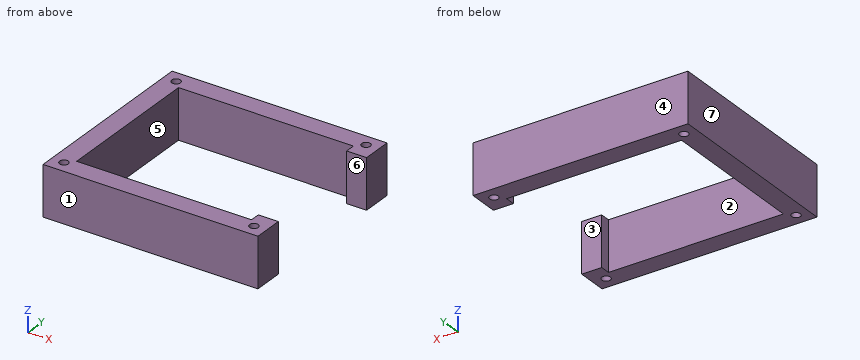
```python
from build123d import *

# Parameters (mm, degrees)
SKETCH_1_W          = 86
SKETCH_1_H          = 76
SKETCH_1_R          = 1.75
SKETCH_1_W_2        = 70
SKETCH_1_H_2        = 60
EXTRUDE_1_DEPTH     = 20
CUT_EXTRUDE_1_REACH = 62.77
SKETCH_2_W          = 8
SKETCH_2_H          = 52


with BuildPart() as part:
    # 草图1 → 凸台-拉伸1 (new body)
    with BuildSketch(Plane.XY):
        Rectangle(SKETCH_1_W, SKETCH_1_H)
        with Locations((-38, 33)):
            Circle(SKETCH_1_R, mode=Mode.SUBTRACT)
        with Locations((38, 33)):
            Circle(SKETCH_1_R, mode=Mode.SUBTRACT)
        with Locations((38, -33)):
            Circle(SKETCH_1_R, mode=Mode.SUBTRACT)
        with Locations((-38, -33)):
            Circle(SKETCH_1_R, mode=Mode.SUBTRACT)
        Rectangle(SKETCH_1_W_2, SKETCH_1_H_2, mode=Mode.SUBTRACT)
    extrude(amount=EXTRUDE_1_DEPTH)

    # 草图2 → 切除-拉伸1 (cut, up to next)
    with BuildSketch(Plane(origin=(0, 0, 0), x_dir=(-1, 0, 0), z_dir=(0, 0, -1)), mode=Mode.PRIVATE) as cut_extrude_1_sk1:
        with Locations((-39, 0)):
            Rectangle(SKETCH_2_W, SKETCH_2_H)
    cut_extrude_1_tool1 = extrude(cut_extrude_1_sk1.sketch, amount=-CUT_EXTRUDE_1_REACH, mode=Mode.PRIVATE) & part.part
    add(cut_extrude_1_tool1.solids().sort_by_distance((39, 0, 0))[0], mode=Mode.SUBTRACT)


solid = part.part
```
CAD build for the part. Positions are in the model's coordinates, mm. Face numbers are marked on the shaded views. A direction names the side the tool comes from. Coordinates: 2 decimals unless noted, no trailing zeros. Write each loop counter-clockwise with the first axis right and the second up, starting at its lowest first coordinate (ties: lowest second). Pieces come first, ordered by that corner, then holes. Notation, with made-up numbers: (-19.75, 76) -> (-3.75, 76) arc R23 ccw to (-3.75, 91) -> close; hole circle Ø4 at (-8, -24.5). An arc over 180 degrees is marked (long way). Return JSON: item names as keys, results as strings. Group by question number.
Q1. Drill centre lines: line 1 (Y direction, x = -38, z = 10); line 2 (Y direction, x = 38, z = 12); line 3 (Y direction, x = -33, z = 9.75). Where is each one in solid material? Low to high.
Q2. Which spindle directions (+Z, -Z, +X, -X, +Y, -Y) get a long thin tool onto all of the face, cutting with end or side? Do the marked faces 1, 2 and 3. Say none if no direction does.
Q3. Flat gauge pins, fed straight in: pin 1 (6 mm diameter, centred on y = -7, z = 11, fed in from +X); pin 2 (3 mm diameter, centred on x = 38, y = 33, fed in from +Z). Where does each tip first touch, or does it go through?
Q4. Cut at B-B, the plane z = 15.5. Give the cut face in (x, y), then the cut area to 3 significant figures.
Q5. Cut at C-C, the plane x = -17. Give the cut face in (y, z), then the cut area to 3 significant figures.
Q6. Cut at A-A, the plane y = 33. Give the cut face in (x, z), then the cut area to 3 significant figures.
Q7. Cut at D-D, the plane x = -38. Give the cut face in (y, z).
Q8. Pull direction Y, two halves, no side cores. Call the marked faces 4, 5, 6 and 7: released by +Y, released by -Y, zero draft, split by the parting line, or undercut.
Returned:
{
 "1": {"line 1": "y = -38 to -34.75, -31.25 to 31.25, 34.75 to 38", "line 2": "y = -38 to -34.75, -31.25 to -26, 26 to 31.25, 34.75 to 38", "line 3": "y = -38 to -30, 30 to 38"},
 "2": {"face 1": "+Z, -Z, +X, -X, -Y", "face 2": "+Z, -Z", "face 3": "+Z, -Z, +X"},
 "3": {"pin 1": "stops at x = -35", "pin 2": "passes through"},
 "4": {"outline": "(-43, -38) -> (43, -38) -> (43, -26) -> (35, -26) -> (35, -30) -> (-35, -30) -> (-35, 30) -> (35, 30) -> (35, 26) -> (43, 26) -> (43, 38) -> (-43, 38) -> close; hole circle Ø3.5 at (-38, -33); hole circle Ø3.5 at (-38, 33); hole circle Ø3.5 at (38, -33); hole circle Ø3.5 at (38, 33)", "area": "1,880 mm2"},
 "5": {"outline": "(-38, 0) -> (-30, 0) -> (-30, 20) -> (-38, 20) -> close; (30, 0) -> (38, 0) -> (38, 20) -> (30, 20) -> close", "area": "320 mm2"},
 "6": {"outline": "(-43, 0) -> (-39.75, 0) -> (-39.75, 20) -> (-43, 20) -> close; (-36.25, 0) -> (36.25, 0) -> (36.25, 20) -> (-36.25, 20) -> close; (39.75, 0) -> (43, 0) -> (43, 20) -> (39.75, 20) -> close", "area": "1,580 mm2"},
 "7": {"outline": "(-38, 0) -> (-34.75, 0) -> (-34.75, 20) -> (-38, 20) -> close; (-31.25, 0) -> (31.25, 0) -> (31.25, 20) -> (-31.25, 20) -> close; (34.75, 0) -> (38, 0) -> (38, 20) -> (34.75, 20) -> close"},
 "8": {"face 4": "released by +Y", "face 5": "undercut", "face 6": "undercut", "face 7": "zero draft"}
}
